Job drawing, mm, ordinate dimensions from the low corner. One solid piece. A direction names the side the tool comes from. Round coordinates to 2 decimals unless told otherwise and drop trailing zeros. Loops run counter-clockwise (first coordinate to the right, second up) from the corner with the lowest first, then second, coordinate; pieces in that order, holes last.
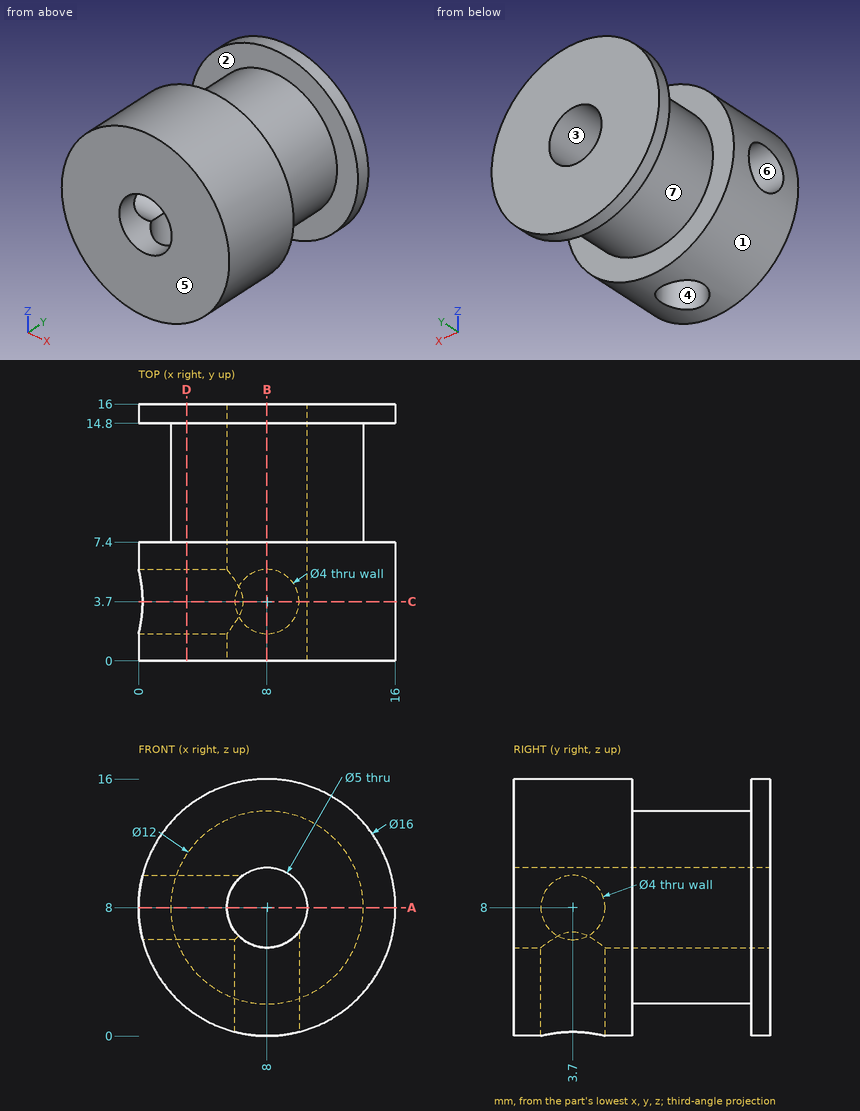
Item 1: 3-axis set-ups, long thin cutter, end or side, ignore diameter. For the marked faces 4, 5, 6 and 7: which of +Z, -Z, +X, -X, +Y, -Y reach the whole face in a straight line?
Answers follow:
face 4: -Z
face 5: +Z, -Z, +X, -X, -Y
face 6: -X
face 7: none
Item 2: Cut at D-D, the plane x = 3. Give the cut face in (y, z) (3 decimals), plus the area to 3 significant figures.
Answers follow:
outline: (0, 1.755) - (7.4, 1.755) - (7.4, 4.683) - (14.8, 4.683) - (14.8, 1.755) - (16, 1.755) - (16, 14.245) - (14.8, 14.245) - (14.8, 11.317) - (7.4, 11.317) - (7.4, 14.245) - (0, 14.245) - close; hole circle Ø4 at (3.7, 8)
area: 144 mm2
Item 3: Cut at C-C, the plane y = 3.7. Give the cut face in (x, z).
Answers follow:
outline: (0.25, 6) arc R8 ccw to (6, 0.25) - (6, 6) - close; (0.25, 10) - (6.5, 10) arc R2.5 cw to (10, 6.5) - (10, 0.25) arc R8 ccw (long way) to start
Item 4: Probe line 1 (Y direction, x = 8, z = 1.5); line 2 (Y direction, x = 7.75, z = 14.75); line 3 (Z direction, x = 8, y = 8.25). List the from-to ranges inside material, lowest first.
Answers follow:
line 1: y = 0 to 1.7, 5.7 to 7.4, 14.8 to 16
line 2: y = 0 to 7.4, 14.8 to 16
line 3: z = 2 to 5.5, 10.5 to 14
Item 5: Two-plate mould, pull along X, no slides. Class the marked faces 1, 2 and 3: released by +X, released by -X, zero draft, split by the parting line, or undercut.
Answers follow:
face 1: split by the parting line
face 2: zero draft
face 3: undercut
Item 6: Flat gauge pins, fed straight in: P1, Ø3, axis at y = 4, z = 6.5, coming from the -X side; P2, Ø4.5, axis at y = 3.7, z = 8, coming from the -X side; P3, Ø1, axis at x = 7, y = 10.5, coming from the +Z side. Where does each tip first touch, or does it go through?
Answers follow:
P1: stops at x = 0.07
P2: stops at x = 0
P3: stops at z = 13.98
Item 7: Cut at A-A, the plane z = 8. Give the cut face in (x, y), plus the area to 3 significant figures.
Answers follow:
outline: (0, 0) - (5.5, 0) - (5.5, 1.7) - (0, 1.7) - close; (0, 5.7) - (5.5, 5.7) - (5.5, 16) - (0, 16) - (0, 14.8) - (2, 14.8) - (2, 7.4) - (0, 7.4) - close; (10.5, 0) - (16, 0) - (16, 7.4) - (14, 7.4) - (14, 14.8) - (16, 14.8) - (16, 16) - (10.5, 16) - close
area: 124 mm2
Item 8: Cut at B-B, the plane x = 8. Give the cut face in (y, z), plus the area to 3 significant figures.
Answers follow:
outline: (0, 0) - (1.7, 0) - (1.7, 5.5) - (0, 5.5) - close; (0, 10.5) - (16, 10.5) - (16, 16) - (14.8, 16) - (14.8, 14) - (7.4, 14) - (7.4, 16) - (0, 16) - close; (5.7, 0) - (7.4, 0) - (7.4, 2) - (14.8, 2) - (14.8, 0) - (16, 0) - (16, 5.5) - (5.7, 5.5) - close
area: 124 mm2
